```python
from build123d import *

# Parameters (mm, degrees)
CROQUIS1_W              = 300
CROQUIS1_H              = 270
SALIENTE_EXTRUIR1_DEPTH = 25.4
VACIADO1_T              = -3


with BuildPart() as part:
    # Croquis1 → Saliente-Extruir1 (new body)
    with BuildSketch(Plane(origin=(0, 0, 0), x_dir=(1, 0, 0), z_dir=(0, 1, 0))):
        Rectangle(CROQUIS1_W, CROQUIS1_H)
    extrude(amount=SALIENTE_EXTRUIR1_DEPTH)

    # Vaciado1
    vaciado1_openings = [part.faces().sort_by_distance(p)[0] for p in [
        (0, 25.4, 0),
    ]]
    offset(amount=VACIADO1_T, openings=vaciado1_openings, kind=Kind.INTERSECTION)


solid = part.part
```
Work out the finished part from the listing and answer in its coordinate system (mm). A direction names the side the tool comes from. Round coordinates to 2 decimals unless told otherwise and drop trailing zeros. Order: outer loops, then holes, each group sorted by start corner. A loop starts at its lowest first (then second) coordinate and runs counter-clockwise, first axis right, second up.
Q1. A tool of negligible diameter and unlimited length cuts with its end or side. For faces 1 (the flat face through (147, 14, 2)), 2 (the flat face through (150, 13, 2)), from which of +Z, -Z, +X, -X, +Y, -Y can it reach the whole face along a straight path? Write none if from no direction.
Solution:
face 1: +Y
face 2: +Z, -Z, +X, +Y, -Y
Q2. A cutting plane is placed at A-A, the plane y = 11.5. Determine the outline of the cut face in (x, z), then the cut area to 3 significant figures.
Solution:
outline: (-150, -135) - (150, -135) - (150, 135) - (-150, 135) - close; hole (-147, -132) - (147, -132) - (147, 132) - (-147, 132) - close
area: 3,380 mm2
Q3. A cutting plane is placed at B-B, the plane x = 4.5. Determine the outline of the cut face in (y, z), then the cut area to 3 significant figures.
Solution:
outline: (0, -135) - (25.4, -135) - (25.4, -132) - (3, -132) - (3, 132) - (25.4, 132) - (25.4, 135) - (0, 135) - close
area: 944 mm2
Q4. Find the intervals of material crossed by line 1 along X through (y, z) = (9, -39.5); line 2 along Z through (x, y) = (100.5, 4.5); line 3 along Y through (x, z) = (-101, -42.5), in increasing order.
Solution:
line 1: x = -150 to -147, 147 to 150
line 2: z = -135 to -132, 132 to 135
line 3: y = 0 to 3
Q5. Given pin 1 Ø1.5 at (x, z) = (86.5, -70.5) entering from -Y, flat-ended and moving along its own axis, determine where the tip first touches the part or whether it passes through.
Solution:
pin 1: stops at y = 0
Q6. The mould has two halves that part along X. Classify faces 3 (the flat face through (-150, 13, 2)), 4 (the flat face through (-2, 13, -135)), 5 (the flat face through (-2, 3, -2)), 6 (the flat face through (-147, 14, 2)): pulls with the +X half, pulls with the -X half, needs draft (parallel to the pull), parting line crosses it, or undercut.
Solution:
face 3: pulls with the -X half
face 4: needs draft
face 5: undercut
face 6: undercut
Q7. A cutting plane is placed at C-C, the plane z = 77. Determine the outline of the cut face in (x, y), then the cut area to 3 significant figures.
Solution:
outline: (-150, 0) - (150, 0) - (150, 25.4) - (147, 25.4) - (147, 3) - (-147, 3) - (-147, 25.4) - (-150, 25.4) - close
area: 1,030 mm2
